Verification items for the finished model (mm, model axes). A direction names the side the tool comes from. Coordinates: 2 decimals unless noted, no trailing zeros. Write each loop counter-clockwise with the first axis right and the second up, starting at its lowest first coordinate (ties: lowest second). Pieces come first, ordered by that corner, then holes. Notation, with made-up numbers: M 11.5,-36 L 34.5,-36 A34 cw 34.5,-4 Z; hole C 6,86.25 d1. An arc over 180 degrees is marked long. Answer in a Markdown table with one row per item.
from build123d import *

# Parameters (mm, degrees)
F0_W     = 10
F0_H     = 170
F1_DEPTH = 37.5
F2_W     = 65
F2_H     = 4.9
F3_DEPTH = 10
F4_W     = 75
F4_H     = 170
F4_W_2   = 65
F4_H_2   = 144.9
F5_DEPTH = 50
F6_W     = 75
F6_H     = 170
F6_W_2   = 25
F6_H_2   = 50
F7_DEPTH = 25


with BuildPart() as f1:
    # F0 (on Right) → F1 (new body, symmetric)
    with BuildSketch(Plane.YZ):
        with Locations((-36.757313, -17.352806)):
            Rectangle(F0_W, F0_H)
    extrude(amount=F1_DEPTH, both=True)

    # F2 (on face) → F3 (cut, through all)
    with BuildSketch(Plane.XZ.offset(41.757313)):
        with Locations((0, 65.097194)):
            Rectangle(F2_W, F2_H)
        with Locations((0, 55.097194)):
            Rectangle(F2_W, F2_H)
        with Locations((0, 45.097194)):
            Rectangle(F2_W, F2_H)
        with Locations((0, 35.097194)):
            Rectangle(F2_W, F2_H)
        with Locations((0, 25.097194)):
            Rectangle(F2_W, F2_H)
        with Locations((0, 15.097194)):
            Rectangle(F2_W, F2_H)
        with Locations((0, 5.097194)):
            Rectangle(F2_W, F2_H)
        with Locations((0, -4.902806)):
            Rectangle(F2_W, F2_H)
        with Locations((0, -14.902806)):
            Rectangle(F2_W, F2_H)
        with Locations((0, -24.902806)):
            Rectangle(F2_W, F2_H)
        with Locations((0, -34.902806)):
            Rectangle(F2_W, F2_H)
        with Locations((0, -44.902806)):
            Rectangle(F2_W, F2_H)
        with Locations((0, -54.902806)):
            Rectangle(F2_W, F2_H)
        with Locations((0, -64.902806)):
            Rectangle(F2_W, F2_H)
        with Locations((0, -74.902806)):
            Rectangle(F2_W, F2_H)
        with Locations((0, -84.902806)):
            Rectangle(F2_W, F2_H)
    extrude(amount=-F3_DEPTH, mode=Mode.SUBTRACT)

    # F4 (on face) → F5 (join)
    with BuildSketch(Plane.XZ.offset(41.757313)):
        with Locations((0, -17.352806)):
            Rectangle(F4_W, F4_H)
        with Locations((0, -14.902806)):
            Rectangle(F4_W_2, F4_H_2, mode=Mode.SUBTRACT)
    extrude(amount=F5_DEPTH)

    # F6 (on face) → F7 (join)
    with BuildSketch(Plane.XZ.offset(91.757313)):
        with Locations((0, -17.352806)):
            Rectangle(F6_W, F6_H)
        with Locations((0, -17.352806)):
            Rectangle(F6_W_2, F6_H_2, mode=Mode.SUBTRACT)
    extrude(amount=F7_DEPTH)


solid = f1.part
1) Sectioned sample at A-A (z = -15). Record the cut outline in (x, y).
Response values:
| item | result |
|---|---|
| outline | M -37.5,-116.76 L -12.5,-116.76 L -12.5,-91.76 L -32.5,-91.76 L -32.5,-31.76 L -37.5,-31.76 Z; M 12.5,-116.76 L 37.5,-116.76 L 37.5,-31.76 L 32.5,-31.76 L 32.5,-91.76 L 12.5,-91.76 Z |
2) Sectioned sample at D-D (x = 27.5). Give the number of separate pieces and of enclosed holes in the cut face, then the cut area to 3 significant figures.
Response values:
| item | result |
|---|---|
| separate pieces | 15 |
| enclosed holes | 0 |
| area | 6,420 mm² |
3) Sectioned sample at B-B (y = -88). Record the cut outline in (x, z).
Response values:
| item | result |
|---|---|
| outline | M -37.5,-102.35 L 37.5,-102.35 L 37.5,67.65 L -37.5,67.65 Z; hole M -32.5,-87.35 L 32.5,-87.35 L 32.5,57.55 L -32.5,57.55 Z |
4) Release check for a two-part mould opening along Z. For faces 1 (the face through (16, -116.757, -16)), 2 (the face through (0, -41.757, -20)), 3 (the face through (0, -37, -77.353)) record: +Z half, -Z half, draft (parallel to the pull), parting line (faces both ways), or undercut.
Response values:
| item | result |
|---|---|
| face 1 | draft |
| face 2 | undercut |
| face 3 | undercut |
5) Sectioned sample at C-C (z = -55). Record the cut outline in (x, y), then the cut area to 4 significant figures.
Response values:
| item | result |
|---|---|
| outline | M -37.5,-116.76 L 37.5,-116.76 L 37.5,-31.76 L 32.5,-31.76 L 32.5,-91.76 L -32.5,-91.76 L -32.5,-31.76 L -37.5,-31.76 Z |
| area | 2,475 mm² |
6) Tool access check on faces 4 (the face through (0, -41.757, 10)), 5 (the face through (0, -37, 47.547)), 6 (the face through (12.5, -104, -18)). Record the directions out of +Z, -Z, +X, -X, +Y, -Y that give a thin tool (end or side, any length) a straight path to the whole face; none if there is none.
Response values:
| item | result |
|---|---|
| face 4 | none |
| face 5 | +Y |
| face 6 | -Y |
7) Thickness scan on L1, parallel to Z at x = 26.5, y = -68; L2, parallel to Y at x = -30, z = 9.5; L3, parallel to X at y = -78.5, z = 11.5. Record the ranges inside material, lowest first. Write a range as [from, to].
Response values:
| item | result |
|---|---|
| L1 | z = [-102.35, -87.35], [57.55, 67.65] |
| L2 | y = [-116.76, -91.76], [-41.76, -31.76] |
| L3 | x = [-37.5, -32.5], [32.5, 37.5] |
8) Depth check by flat-ended pin: pin 1 (1.5 mm diameter, centred on x = -5, z = 3.5, fed in from -Y); pin 2 (2.5 mm diameter, centred on x = 7, z = -31, fed in from -Y). Enter the tip coordinate at first touch or a pass-through.
Response values:
| item | result |
|---|---|
| pin 1 | passes through |
| pin 2 | stops at y = -41.76 |
